Input: part model. Units: mm. Frame: model coordinates. Face numbers are marked on the shaded views. A direction names the side the tool comes from. Coordinates: 2 decimals unless noted, no trailing zeros. Order: outer loops, then holes, each group sorted by start corner. A loop starts at its lowest first (then second) coordinate and runs counter-clockwise, first axis right, second up.
from build123d import *

# Parameters (mm, degrees)
ESQUISSE1_R             = 12
BOSS_EXTRU_1_DEPTH      = 20.5
ESQUISSE2_R             = 2.5
BOSS_EXTRU_2_DEPTH      = 3.5
ESQUISSE3_R             = 1.8
ENL_V_MAT_EXTRU_1_DEPTH = 3
ESQUISSE4_R             = 2.5
BOSS_EXTRU_3_DEPTH      = 6.5
ESQUISSE5_R             = 5
BOSS_EXTRU_4_DEPTH      = 14
CONG_1_R                = 1


with BuildPart() as part:
    # Esquisse1 → Boss.-Extru.1 (new body)
    with BuildSketch(Plane.XY):
        Circle(ESQUISSE1_R)
    extrude(amount=BOSS_EXTRU_1_DEPTH)

    # Esquisse2 → Boss.-Extru.2 (add)
    with BuildSketch(Plane.XY.offset(20.5)):
        Circle(ESQUISSE2_R)
    extrude(amount=BOSS_EXTRU_2_DEPTH)

    # Esquisse3 → Enlèv. mat.-Extru.1 (cut)
    with BuildSketch(Plane.XY.offset(20.5)):
        with Locations((0, 9)):
            Circle(ESQUISSE3_R)
        with Locations((-7.794228634, -4.5)):
            Circle(ESQUISSE3_R)
        with Locations((7.794228634, -4.5)):
            Circle(ESQUISSE3_R)
    extrude(amount=-ENL_V_MAT_EXTRU_1_DEPTH, mode=Mode.SUBTRACT)

    # Esquisse4 → Boss.-Extru.3 (add)
    with BuildSketch(Plane.XY.offset(24)):
        Circle(ESQUISSE4_R)
    extrude(amount=BOSS_EXTRU_3_DEPTH)

    # Esquisse5 → Boss.-Extru.4 (add)
    with BuildSketch(Plane(origin=(0, 0, 0), x_dir=(1, 0, 0), z_dir=(0, 1, 0))):
        with Locations((0, -8)):
            Circle(ESQUISSE5_R)
    extrude(amount=-BOSS_EXTRU_4_DEPTH)

    # Congé1
    cong_1_edges = [part.edges().sort_by_distance(p)[0] for p in [
        (-5, -14, 8),
    ]]
    fillet(cong_1_edges, radius=CONG_1_R)


solid = part.part
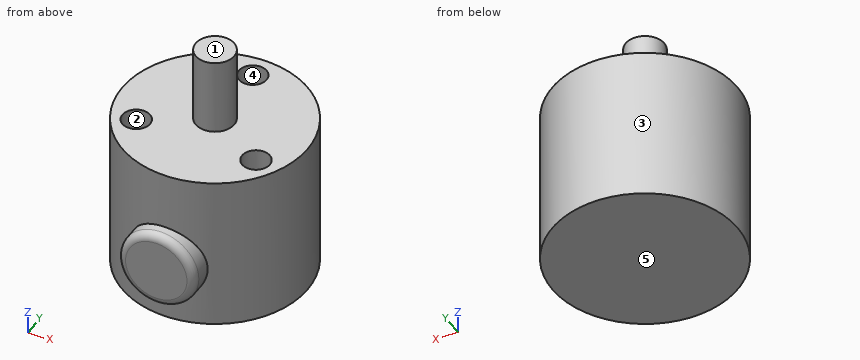
Item 1: Access query for the marked faces 1 and 2. Directions: +Z, -Z, +X, -X, +Y, -Y. A direction counts if a zero-diameter tool reaches every point of the face in a straight line with its end or side. Return the directions, or none.
Response values:
face 1: +Z, +X, -X, +Y, -Y
face 2: +Z
Item 2: Draft query along Y for the marked faces 3, 4 and 5. Return one class per face: pulls with the +Y half, pulls with the -Y half, needs draft (parallel to the pull), parting line crosses it, or undercut.
Response values:
face 3: parting line crosses it
face 4: undercut
face 5: needs draft
Item 3: Ray query, probe 1 along Y at (x, z) = (0, 19.8); probe 2 along Z at (x, y) = (6.5, -9.75); probe 3 along Z at (x, y) = (-8, -3). Return the intervals inside material, ascending.
Response values:
probe 1: y = -12 to 7.2, 10.8 to 12
probe 2: z = 0 to 20.5
probe 3: z = 0 to 17.5
Item 4: Cut plane B-B on y = 0. Return loops of the section in (x, z).
Response values:
outline: (-12, 0) - (12, 0) - (12, 20.5) - (2.5, 20.5) - (2.5, 30.5) - (-2.5, 30.5) - (-2.5, 20.5) - (-12, 20.5) - close
Item 5: Cut plane A-A on x = 0. Return loops of the section in (y, z), then the cut area to 3 significant figures.
Response values:
outline: (-14, 4) arc R1 ccw to (-13, 3) - (-12, 3) - (-12, 0) - (12, 0) - (12, 20.5) - (10.8, 20.5) - (10.8, 17.5) - (7.2, 17.5) - (7.2, 20.5) - (2.5, 20.5) - (2.5, 30.5) - (-2.5, 30.5) - (-2.5, 20.5) - (-12, 20.5) - (-12, 13) - (-13, 13) arc R1 ccw to (-14, 12) - close
area: 551 mm2
Item 6: Cut plane C-C on z = 8. Return loops of the section in (x, y), then the cut area to 3 significant figures.
Response values:
outline: (-5, -13) arc R1 ccw to (-4, -14) - (4, -14) arc R1 ccw to (5, -13) - (5, -10.91) arc R12 ccw (long way) to (-5, -10.91) - close
area: 476 mm2
Item 7: Pin query (flat end, axial travel): pin 1 Ø3 at (x, y) = (0, 9) entering from -Z; pin 2 Ø3 at (x, y) = (7.5, -4) entering from +Z; pin 3 Ø5 at (y, z) = (-6.5, 9.5) entering from -X; pin 4 Ø12 at (x, z) = (0.5, 27) entering from +Y. Return the tip coordinate at first contact, or that it passes through.
Response values:
pin 1: stops at z = 0
pin 2: stops at z = 20.5
pin 3: stops at x = -11.31
pin 4: stops at y = 2.5
Item 8: Cut plane D-D on x = -7. Return loops of the section in (y, z).
Response values:
outline: (-9.75, 0) - (9.75, 0) - (9.75, 20.5) - (-2.88, 20.5) - (-2.88, 17.5) - (-6.12, 17.5) - (-6.12, 20.5) - (-9.75, 20.5) - close
